from build123d import *

# Parameters (mm, degrees)
F1_DEPTH = 5
F4_DEPTH = 5


# Not quite as in the source:
# - a feature of the source that left no trace in its solid (it failed there, or was rolled back) is left out


with BuildPart() as f1:
    # F0 (on Top) → F1 (new body)
    with BuildSketch(Plane.XY):
        with BuildLine():
            Line((67.2432569916, 68.9932702117), (-49.1140455478, 60.1726392496))
            ThreePointArc((-49.1140455478, 60.1726392496), (-53.2152003045, 59.1119075124), (-56.692252409, 56.692252409))
            Line((-56.692252409, 56.692252409), (-36.0883415168, 36.0883415168))
            Line((-36.0883415168, 36.0883415168), (-34.2875776013, 34.2875776013))
            ThreePointArc((-34.2875776013, 34.2875776013), (-31.969542865, 35.9006810036), (-29.2354396938, 36.607835495))
            Line((-29.2354396938, 36.607835495), (69.1329955604, 44.0647947641))
            Line((69.1329955604, 44.0647947641), (67.2432569916, 68.9932702117))
        make_face()
    extrude(amount=F1_DEPTH)

    # F0 (on Top) → F4 (join)
    with BuildSketch(Plane.XY):
        with BuildLine():
            Line((-36.0883415168, 36.0883415168), (-56.692252409, 56.692252409))
            ThreePointArc((-56.692252409, 56.692252409), (-59.1119075124, 53.2152003045), (-60.1726392496, 49.1140455478))
            Line((-60.1726392496, 49.1140455478), (-68.9932702117, -67.2432569916))
            Line((-68.9932702117, -67.2432569916), (-44.0647947641, -69.1329955604))
            Line((-44.0647947641, -69.1329955604), (-36.607835495, 29.2354396938))
            ThreePointArc((-36.607835495, 29.2354396938), (-35.9006810036, 31.969542865), (-34.2875776013, 34.2875776013))
            Line((-34.2875776013, 34.2875776013), (-36.0883415168, 36.0883415168))
        make_face()
    extrude(amount=F4_DEPTH)


solid = f1.part
Read the model definition and answer for the solid it produces. Units are mm, in the model's axes. Coordinates: 2 decimals unless noted, no trailing zeros. Write each loop counter-clockwise with the first axis right and the second up, starting at its lowest first coordinate (ties: lowest second). Pieces come first, ordered by that corner, then holes. Notation, with made-up numbers: (40.25, 0.5) -> (98.25, 0.5) arc R34 ccw to (98.25, 31.5) -> close; hole circle Ø1 at (75.25, 7). An arc over 180 degrees is marked (long way). Return JSON: item names as keys, results as strings.
(1) Each of these flat-tipped pins is pushed along its axis until it touches: P1, Ø1, axis at y = -20, z = 3.5, coming from the -X side; P2, Ø1.5, axis at x = 31.5, z = 1.5, coming from the +Y side; P3, Ø1.5, axis at x = 46, z = 1.5, coming from the -Y side; P4, Ø1.5, axis at x = -38.5, y = -9.5, coming from the -Z side. Where does it stop, or does it pass through?
Answers below:
{"P1": "x = -65.45", "P2": "y = 66.34", "P3": "y = 42.25", "P4": "through"}
(2) Consider line 1 along X through (y, z) = (21, 0.2); line 2 along X through (y, z) = (-2.5, 2.75); line 3 along Y through (x, z) = (37, 2.55). Determine where each line is inside the solid, lowest interval first. Write a range as from..to.
Answers below:
{"line 1": "-62.3..-37.23", "line 2": "-64.09..-39.01", "line 3": "41.63..66.7"}
(3) The part is cut by section A-A on z = 1.4. Give the vertices of the cut face in (x, y), then the cut area to 3 significant figures.
Answers below:
{"outline": "(-68.99, -67.24) -> (-44.06, -69.13) -> (-36.61, 29.24) arc R8 cw to (-29.24, 36.61) -> (69.13, 44.06) -> (67.24, 68.99) -> (-49.11, 60.17) arc R12 ccw to (-60.17, 49.11) -> close", "area": "5,800 mm^2"}
(4) The part is cut by section B-B on y = 55. Give the vertices of the cut face in (x, z), then the cut area to 3 significant figures.
Answers below:
{"outline": "(-58.1, 0) -> (68.3, 0) -> (68.3, 5) -> (-58.1, 5) -> close", "area": "632 mm^2"}
(5) The part is cut by section C-C on x = 1. Give the vertices of the cut face in (y, z), then the cut area to 3 significant figures.
Answers below:
{"outline": "(38.9, 0) -> (63.97, 0) -> (63.97, 5) -> (38.9, 5) -> close", "area": "125 mm^2"}
